The model under review builds one solid part; all positions refer to its coordinate system, in mm. Face numbers are marked on the shaded views. A direction names the side the tool comes from. Give positions to 0.01 mm unless a question says otherwise; leave off trailing zeros. Loops run counter-clockwise (first coordinate to the right, second up) from the corner with the lowest first, then second, coordinate; pieces in that order, holes last. Notation, with made-up numbers: M -2,87 L 13,87 A19 ccw 13,111 Z; hole C 30,-9.75 d10. An arc over 180 degrees is marked long. Write item = value, one per line. Start each with the question number.
1. For the marked faces 1, 2 and 3, list the 3-axis set-ups (+Z, -Z, +X, -X, +Y, -Y) from which the entire face can be reached by the end or side of a thin tool; tool diameter is ignored.
2. We need section B-B on y = 32. Give the boundary of the cut face in (x, z).
3. Wall thickness on line 1 along X through (y, z) = (6, 0); line 2 along Z through (x, y) = (1.5, 19.5); line 3 along Z through (x, y) = (-2, 9): over which ranges is each line inside the solid? List them lowest first. Write a range as from..to.
4. We need section D-D on y = 6. Give the boundary of the cut face in (x, z), then the cut area to 3 significant figures.
5. We need section A-A on x = 0. Give the boundary of the cut face in (y, z), then the cut area to 3 significant figures.
6. Draft analysis for pull direction Z (two halves, no side actions). For the marked faces 4, 5 and 6, state which applies: pulls with the +Z half, pulls with the -Z half, needs draft (parallel to the pull), parting line crosses it, or undercut.
7. We need section C-C on z = 0. Give the boundary of the cut face in (x, y).
8. For pin 1 (1 mm diameter, centred on y = 8, z = 5.5, fed in from -X); pin 2 (4.5 mm diameter, centred on x = 3, y = 31, fed in from +Z); pin 3 (2 mm diameter, centred on y = 9.5, z = 9, fed in from -X), all flat-tipped, find the tip position at first contact; note any pin that passes through.
from build123d import *

# Parameters (mm, degrees)
SKETCH1_R           = 6.5
SKETCH1_R_2         = 4.08
BOSS_EXTRUDE1_DEPTH = 20
SKETCH2_R           = 15
BOSS_EXTRUDE2_DEPTH = 2
SKETCH3_R           = 15
SKETCH3_W           = 16
SKETCH3_H           = 16
BOSS_EXTRUDE3_DEPTH = 15
BOSS_EXTRUDE4_START = 20
SKETCH4_R           = 15
SKETCH4_R_2         = 6.5
BOSS_EXTRUDE4_DEPTH = 20
SKETCH6_R           = 1
CUT_EXTRUDE1_DEPTH  = 24
CUT_EXTRUDE2_START  = 10
SKETCH8_R           = 3
SKETCH8_R_2         = 1
CUT_EXTRUDE2_DEPTH  = 10
CHAMFER1_SIZE       = 2


with BuildPart() as part:
    # Sketch1 → Boss-Extrude1 (new body)
    with BuildSketch(Plane(origin=(0, 0, 0), x_dir=(1, 0, 0), z_dir=(0, 1, 0))):
        with Locations(Location((0, 0, 0), (0, 0, 270))):
            Circle(SKETCH1_R)
        with Locations(Location((0, 0, 0), (0, 0, 270))):
            Circle(SKETCH1_R_2, mode=Mode.SUBTRACT)
    extrude(amount=BOSS_EXTRUDE1_DEPTH)

    # Sketch2 → Boss-Extrude2 (add)
    with BuildSketch(Plane(origin=(0, 20, 0), x_dir=(1, 0, 0), z_dir=(0, 1, 0))):
        with Locations(Location((0, 0, 0), (0, 0, 270))):
            Circle(SKETCH2_R)
    extrude(amount=BOSS_EXTRUDE2_DEPTH)

    # Sketch3 → Boss-Extrude3 (add)
    with BuildSketch(Plane(origin=(0, 22, 0), x_dir=(1, 0, 0), z_dir=(0, 1, 0))):
        with Locations(Location((0, 0, 0), (0, 0, 270))):
            Circle(SKETCH3_R)
        Rectangle(SKETCH3_W, SKETCH3_H, mode=Mode.SUBTRACT)
    extrude(amount=BOSS_EXTRUDE3_DEPTH)

    # Sketch4 → Boss-Extrude4 (add)
    with BuildSketch(Plane.XZ.offset(-20).offset(BOSS_EXTRUDE4_START)):
        with Locations(Location((0, 0, 0), (0, 0, 90))):
            Circle(SKETCH4_R)
        Circle(SKETCH4_R_2, mode=Mode.SUBTRACT)
    extrude(amount=-BOSS_EXTRUDE4_DEPTH)

    # Sketch6 → Cut-Extrude1 (cut)
    with BuildSketch(Plane.XY):
        with Locations(Location((0, 6, 0), (0, 0, 90))):
            Circle(SKETCH6_R)
    extrude(amount=-CUT_EXTRUDE1_DEPTH, mode=Mode.SUBTRACT)

    # Sketch8 → Cut-Extrude2 (cut)
    with BuildSketch(Plane.XY.offset(-16.5).offset(CUT_EXTRUDE2_START)):
        with Locations(Location((0, 6, 0), (0, 0, 90))):
            Circle(SKETCH8_R)
        with Locations((0, 6)):
            Circle(SKETCH8_R_2, mode=Mode.SUBTRACT)
    extrude(amount=-CUT_EXTRUDE2_DEPTH, mode=Mode.SUBTRACT)

    # Chamfer1
    chamfer1_edges = [part.edges().sort_by_distance(p)[0] for p in [
        (0, 0, -4.08),
    ]]
    chamfer(chamfer1_edges, length=CHAMFER1_SIZE)


solid = part.part
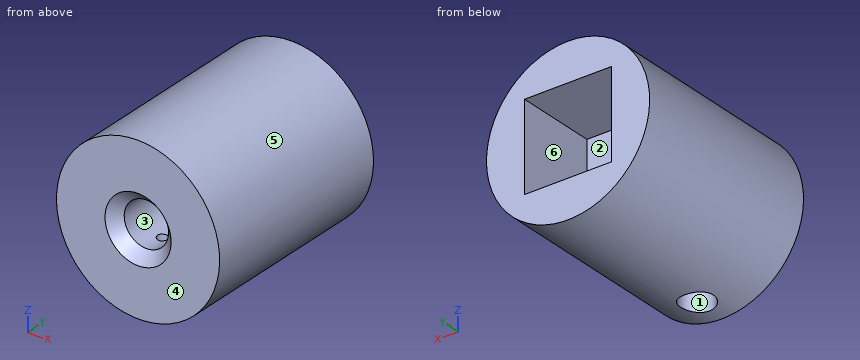
Final values:
q1.face_1 = -Z
q1.face_2 = +Y
q1.face_3 = -Y
q2.outline = C 0,0 d30; hole M -8,-8 L 8,-8 L 8,8 L -8,8 Z
q3.line_1 = -15..-4.08, 4.08..15
q3.line_2 = -14.92..-3.79, 3.79..14.92
q3.line_3 = -14.87..-3.56, 3.56..14.87
q4.outline = M -3,-14.7 L -3,-6.5 L -1,-6.5 L -1,-3.96 A4.08 cw long 1,-3.96 L 1,-6.5 L 3,-6.5 L 3,-14.7 A15 ccw long Z
q4.area = 599 mm²
q5.outline = M 0,-15 L 3,-15 L 3,-6.5 L 5,-6.5 L 5,-4.08 L 2,-4.08 L 0,-6.08 Z; M 0,6.08 L 2,4.08 L 20,4.08 L 20,-4.08 L 7,-4.08 L 7,-6.5 L 9,-6.5 L 9,-15 L 37,-15 L 37,-8 L 22,-8 L 22,8 L 37,8 L 37,15 L 0,15 Z
q5.area = 647 mm²
q6.face_4 = needs draft
q6.face_5 = parting line crosses it
q6.face_6 = undercut
q7.outline = M -15,0 L -6.08,0 L -4.08,2 L -4.08,20 L 4.08,20 L 4.08,2 L 6.08,0 L 15,0 L 15,37 L 8,37 L 8,22 L -8,22 L -8,37 L -15,37 Z
q8.pin_1 = -14.14
q8.pin_2 = 14.98
q8.pin_3 = -12.69
